Geometry: final body of the model. Coordinates: model frame, mm. Coordinates: 2 decimals unless noted, no trailing zeros. Loops run counter-clockwise (first coordinate to the right, second up) from the corner with the lowest first, then second, coordinate; pieces in that order, holes last. Notation, with made-up numbers: (-14.5, 76) - (5.5, 76) arc R17 cw to (5.5, 81) - close; hole circle Ø6 at (62.5, 43). An arc over 180 degrees is marked (long way). Put each result on its own line as item: value. Start each with the question number.
1) Material intervals for line 1 along X through (y, z) = (28.2, 41.5); line 2 along Y through (x, z) = (1, 108); line 3 along Y through (x, z) = (-15, 115), sorted ascending. Write a range as from..to.
2) Section B-B on z = 41.5. Output: boundary loops of the cut face in (x, y).
3) Section A-A on x = 4.5. Output: boundary loops of the cut face in (y, z), and give its area (3 significant figures).
4) Section D-D on x = 17. Output: boundary loops of the cut face in (y, z), and give its area (3 significant figures).
5) Contact query for flat-ended pins moving along their axis: pin 1 Ø0.9 at (x, y) = (15.5, 28.5) entering from +Z; pin 2 Ø10 at (x, z) = (-20.5, 31) entering from +Y; pin 3 Ø2 at (y, z) = (8.5, 35.5) entering from -X. Output: stop coordinate, or through.
6) Section C-C on y = 10. Output: boundary loops of the cut face in (x, z).
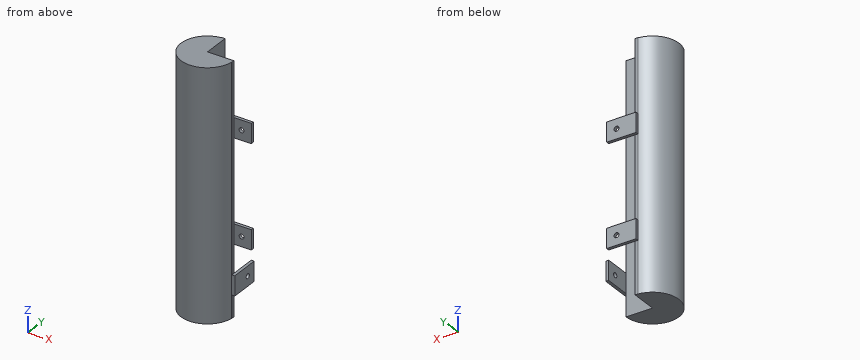
```python
from build123d import *

# Parameters (mm, degrees)
BOSS_EXTRUDE1_DEPTH  = 126.5
SKETCH12_W           = 20
SKETCH12_H           = 30
BOSS_EXTRUDE6_DEPTH  = 3
CUT_EXTRUDE3_REACH   = 143.366
SKETCH13_R           = 2.5
SKETCH17_W           = 30
SKETCH17_H           = 20
BOSS_EXTRUDE10_DEPTH = 3
CUT_EXTRUDE5_REACH   = 143.957
SKETCH18_R           = 2.5


with BuildPart() as part:
    # Sketch4 → Boss-Extrude1 (new, symmetric)
    with BuildSketch(Plane.XY):
        with BuildLine():
            Line((0, 0), (27, 0))
            Line((27, 0), (27, -3))
            Line((27, -3), (26.800082477, -3))
            ThreePointArc((26.800082477, -3), (-19.135504983, -19.08508544), (-3, 26.83281573))
            Line((-3, 26.83281573), (-3, 27))
            Line((-3, 27), (0, 27))
            Line((0, 27), (0, 0))
        make_face()
    extrude(amount=BOSS_EXTRUDE1_DEPTH, both=True)

    # Sketch12 → Boss-Extrude6 (add)
    with BuildSketch(Plane(origin=(27, 0, 0), x_dir=(0, 0, -1), z_dir=(1, 0, 0))):
        with Locations((93.5, 12)):
            Rectangle(SKETCH12_W, SKETCH12_H)
    extrude(amount=BOSS_EXTRUDE6_DEPTH)

    # Sketch13 → Cut-Extrude3 (cut, up to next)
    with BuildSketch(Plane(origin=(30, 0, 0), x_dir=(0, 0, -1), z_dir=(1, 0, 0)), mode=Mode.PRIVATE) as cut_extrude3_sk1:
        with Locations((93.5, 17)):
            Circle(SKETCH13_R)
    cut_extrude3_tool1 = extrude(cut_extrude3_sk1.sketch, amount=-CUT_EXTRUDE3_REACH, mode=Mode.PRIVATE) & part.part
    add(cut_extrude3_tool1.solids().sort_by_distance((30, 17, -93.5))[0], mode=Mode.SUBTRACT)

    # Sketch17 → Boss-Extrude10 (add)
    with BuildSketch(Plane(origin=(0, 27, 0), x_dir=(1, 0, 0), z_dir=(0, 1, 0))):
        with Locations((12, 63.5)):
            Rectangle(SKETCH17_W, SKETCH17_H)
        with Locations((12, -41.5)):
            Rectangle(SKETCH17_W, SKETCH17_H)
    extrude(amount=BOSS_EXTRUDE10_DEPTH)

    # Sketch18 → Cut-Extrude5 (cut, up to next)
    with BuildSketch(Plane(origin=(0, 30, 0), x_dir=(1, 0, 0), z_dir=(0, 1, 0)), mode=Mode.PRIVATE) as cut_extrude5_sk1:
        with Locations(Location((17, 63.5, 0), (0, 0, 270))):
            Circle(SKETCH18_R)
    cut_extrude5_tool1 = extrude(cut_extrude5_sk1.sketch, amount=-CUT_EXTRUDE5_REACH, mode=Mode.PRIVATE) & part.part
    # Sketch18 → Cut-Extrude5 (cut, up to next)
    with BuildSketch(Plane(origin=(0, 30, 0), x_dir=(1, 0, 0), z_dir=(0, 1, 0)), mode=Mode.PRIVATE) as cut_extrude5_sk2:
        with Locations(Location((17, -41.5, 0), (0, 0, 270))):
            Circle(SKETCH18_R)
    cut_extrude5_tool2 = extrude(cut_extrude5_sk2.sketch, amount=-CUT_EXTRUDE5_REACH, mode=Mode.PRIVATE) & part.part
    add(cut_extrude5_tool1.solids().sort_by_distance((17, 30, -63.5))[0], mode=Mode.SUBTRACT)
    add(cut_extrude5_tool2.solids().sort_by_distance((17, 30, 41.5))[0], mode=Mode.SUBTRACT)


solid = part.part
```
Answer block:
1. line 1: x = -3..14.5, 19.5..27
1. line 2: y = -26.98..0
1. line 3: y = -22.48..22.47
2. outline: (-3, 26.83) arc R27 ccw (long way) to (26.8, -3) - (27, -3) - (27, 0) - (0, 0) - (0, 27) - (14.5, 27) - (14.5, 30) - (-3, 30) - close; (19.5, 27) - (27, 27) - (27, 30) - (19.5, 30) - close
3. outline: (-26.62, -126.5) - (0, -126.5) - (0, 126.5) - (-26.62, 126.5) - close; (27, -73.5) - (30, -73.5) - (30, -53.5) - (27, -53.5) - close; (27, 31.5) - (30, 31.5) - (30, 51.5) - (27, 51.5) - close
3. area: 6,850 mm²
4. outline: (-20.95, -126.5) - (0, -126.5) - (0, 126.5) - (-20.95, 126.5) - close; (27, -73.5) - (30, -73.5) - (30, -66) - (27, -66) - close; (27, -61) - (30, -61) - (30, -53.5) - (27, -53.5) - close; (27, 31.5) - (30, 31.5) - (30, 39) - (27, 39) - close; (27, 44) - (30, 44) - (30, 51.5) - (27, 51.5) - close
4. area: 5,390 mm²
5. pin 1: stops at z = 51.5
5. pin 2: stops at y = 22.13
5. pin 3: stops at x = -25.97
6. outline: (-25.11, -126.5) - (0, -126.5) - (0, 126.5) - (-25.11, 126.5) - close; (27, -103.5) - (30, -103.5) - (30, -83.5) - (27, -83.5) - close
